from build123d import *

# Parameters (mm, degrees)
SKETCH2_W           = 55
SKETCH2_H           = 115
BOSS_EXTRUDE1_DEPTH = 5
SKETCH5_W           = 50
SKETCH5_H           = 50
SKETCH5_W_2         = 40
SKETCH5_H_2         = 40
SWEEP2_START        = -22.5
SWEEP2_DEPTH        = 50
SWEEP2_2_DEPTH      = 5
SWEEP2_START_2      = 22.5
SWEEP2_3_DEPTH      = 5
SKETCH11_R          = 12.5
CUT_EXTRUDE2_DEPTH  = 25
SKETCH12_R          = 12.5
CUT_EXTRUDE3_DEPTH  = 25
SKETCH13_W          = 2.5
SKETCH13_H          = 115
BOSS_EXTRUDE2_DEPTH = 50
SKETCH15_W          = 2.5
SKETCH15_H          = 115
BOSS_EXTRUDE3_DEPTH = 50
SKETCH14_R          = 7
CUT_EXTRUDE4_DEPTH  = 2185.475051357


# Read off the part's stored shape, not the designer's step: Sweep2
with BuildPart() as part:
    # Sketch2 → Boss-Extrude1 (new body)
    with BuildSketch(Plane(origin=(0, 0, 0), x_dir=(1, 0, 0), z_dir=(0, 1, 0))):
        Rectangle(SKETCH2_W, SKETCH2_H)
    extrude(amount=-BOSS_EXTRUDE1_DEPTH)

    # Sweep1: sweep along a path in Sketch7
    with BuildLine(Plane(origin=(0, 0, 0), x_dir=(0, 0, -1), z_dir=(1, 0, 0))) as sweep1_path:
        Line((-2.5, 0), (-2.5, 1930))
    # Sketch5 → Sweep1 (sweep)
    with BuildSketch(Plane(origin=(0, 0, 0), x_dir=(1, 0, 0), z_dir=(0, 1, 0))):
        with Locations((0, -2.5)):
            Rectangle(SKETCH5_W, SKETCH5_H)
        with Locations((0, -2.5)):
            Rectangle(SKETCH5_W_2, SKETCH5_H_2, mode=Mode.SUBTRACT)
    sweep(path=sweep1_path.line)

    # Sweep2 outline → Sweep2 (add)
    with BuildSketch(Plane.XY.offset(SWEEP2_START)):
        with BuildLine():
            ThreePointArc((125, 2080), (18.933982822, 2036.066017178), (-25, 1930))
            Line((-25, 1930), (-20, 1930))
            ThreePointArc((-20, 1930), (22.469516728, 2032.530483272), (125, 2075))
            Line((125, 2075), (305, 2075))
            Line((305, 2075), (305, 2080))
            Line((305, 2080), (125, 2080))
        make_face()
        with BuildLine():
            ThreePointArc((125, 2035), (50.753787975, 2004.246212025), (20, 1930))
            Line((20, 1930), (25, 1930))
            ThreePointArc((25, 1930), (54.289321881, 2000.710678119), (125, 2030))
            Line((125, 2030), (305, 2030))
            Line((305, 2030), (305, 2035))
            Line((305, 2035), (125, 2035))
        make_face()
    extrude(amount=SWEEP2_DEPTH)

    # Sweep2 2 outline → Sweep2 2 (add)
    with BuildSketch(Plane.XY.offset(SWEEP2_START)):
        with BuildLine():
            ThreePointArc((125, 2075), (22.469516728, 2032.530483272), (-20, 1930))
            Line((-20, 1930), (20, 1930))
            ThreePointArc((20, 1930), (50.753787975, 2004.246212025), (125, 2035))
            Line((125, 2035), (305, 2035))
            Line((305, 2035), (305, 2075))
            Line((305, 2075), (125, 2075))
        make_face()
    extrude(amount=SWEEP2_2_DEPTH)

    # Sweep2 3 outline → Sweep2 3 (add)
    with BuildSketch(Plane.XY.offset(SWEEP2_START_2)):
        with BuildLine():
            ThreePointArc((125, 2075), (22.469516728, 2032.530483272), (-20, 1930))
            Line((-20, 1930), (20, 1930))
            ThreePointArc((20, 1930), (50.753787975, 2004.246212025), (125, 2035))
            Line((125, 2035), (305, 2035))
            Line((305, 2035), (305, 2075))
            Line((305, 2075), (125, 2075))
        make_face()
    extrude(amount=SWEEP2_3_DEPTH)

    # Mirror1: part across plane


with BuildPart() as part_1:
    add(part.part)
    add(part.part.mirror(Plane(origin=(305, 2055, 0), x_dir=(0, 0, 1), z_dir=(1, 0, 0))))

    # Sketch11 → Cut-Extrude2 (cut)
    with BuildSketch(Plane.XZ.offset(-2030)):
        with Locations((395, 2.5)):
            Circle(SKETCH11_R)
    extrude(amount=-CUT_EXTRUDE2_DEPTH, mode=Mode.SUBTRACT)

    # Sketch12 → Cut-Extrude3 (cut)
    with BuildSketch(Plane.XZ.offset(-2030)):
        with Locations((395, 2.5)):
            Circle(SKETCH12_R)
        with Locations(Location((215, 2.5, 0), (0, 0, 180))):
            Circle(SKETCH12_R)
    extrude(amount=-CUT_EXTRUDE3_DEPTH, mode=Mode.SUBTRACT)

    # Sketch13 → Boss-Extrude2 (add)
    with BuildSketch(Plane.XZ.offset(5)):
        with Locations((-26.25, 0)):
            Rectangle(SKETCH13_W, SKETCH13_H)
    extrude(amount=BOSS_EXTRUDE2_DEPTH)

    # Sketch15 → Boss-Extrude3 (add)
    with BuildSketch(Plane.XZ.offset(5)):
        with Locations((636.25, 0)):
            Rectangle(SKETCH15_W, SKETCH15_H)
    extrude(amount=BOSS_EXTRUDE3_DEPTH)

    # Sketch14 → Cut-Extrude4 (cut, through all)
    with BuildSketch(Plane.ZY.offset(27.5)):
        with Locations((-45, -27.5)):
            Circle(SKETCH14_R)
        with Locations((45, -27.5)):
            Circle(SKETCH14_R)
    extrude(amount=-CUT_EXTRUDE4_DEPTH, mode=Mode.SUBTRACT)


solid = part_1.part
The listing builds one solid part. Answer for the finished solid, in the listing's coordinates (mm). A direction names the side the tool comes from. Coordinates: 2 decimals unless noted, no trailing zeros. Loops run counter-clockwise (first coordinate to the right, second up) from the corner with the lowest first, then second, coordinate; pieces in that order, holes last. Notation, with made-up numbers: M 28,42.5 L 34,42.5 A20 cw 34,78.5 Z; hole C 33.25,49 d10. An arc over 180 degrees is marked long. Answer in a Markdown table with one row per item.
1) Determine the mould class of faces 1 (the cylindrical face through (20.11, 2037.23, 2.15)), 2 (the cylindrical face through (21.35, 2031.4, 2.22)), 3 (the flat face through (308, 2030, 2)) for opening direction Y: released by +Y, released by -Y, zero draft, split by the parting line, or undercut.
Answers below:
| item | result |
|---|---|
| face 1 | released by +Y |
| face 2 | undercut |
| face 3 | released by -Y |
2) Find section A-A (y = 999). Determine the outline of the cut face in (x, z), then the cut area to 3 significant figures.
Answers below:
| item | result |
|---|---|
| outline | M -25,-22.5 L 25,-22.5 L 25,27.5 L -25,27.5 Z; M 585,-22.5 L 635,-22.5 L 635,27.5 L 585,27.5 Z; hole M -20,-17.5 L 20,-17.5 L 20,22.5 L -20,22.5 Z; hole M 590,-17.5 L 630,-17.5 L 630,22.5 L 590,22.5 Z |
| area | 1,800 mm^2 |
3) Given pin 1 (20 mm diameter, centred on y = 571.5, z = -7.5, fed in from +X); pin 2 (12 mm diameter, centred on x = 616, z = -3, fed in from +Y); pin 3 (8.5 mm diameter, centred on y = -27.5, z = 45, fed in from -X); pin 4 (3 mm diameter, centred on x = 354, z = 17, fed in from -Y), each flat-ended and moving along its own axis, determine where each tip first touches the part or whether it passes through.
Answers below:
| item | result |
|---|---|
| pin 1 | x = 635 |
| pin 2 | y = 2012.92 |
| pin 3 | through |
| pin 4 | y = 2030 |
4) Find the intervals of material crossed by probe 1 along X at (y, z) = (1484, -8); probe 2 along Y at (x, z) = (-26.6, -45); probe 3 along X at (y, z) = (1209, -19), in increasing order.
Answers below:
| item | result |
|---|---|
| probe 1 | -25 to -20, 20 to 25, 585 to 590, 630 to 635 |
| probe 2 | -55 to -34.5, -20.5 to 0 |
| probe 3 | -25 to 25, 585 to 635 |
5) Find section C-C (x = 527.5). Determine the outline of the cut face in (y, z).
Answers below:
| item | result |
|---|---|
| outline | M 2020.52,-22.5 L 2073.85,-22.5 L 2073.85,27.5 L 2020.52,27.5 Z; hole M 2026.01,-17.5 L 2068.63,-17.5 L 2068.63,22.5 L 2026.01,22.5 Z |
6) Which of the six approach directions +Z, -Z, +X, -X, +Y, -Y give full straight-line access (tool end or side, diameter ignored) to faces 4 (the flat face through (590, 979, 2)), 5 (the flat face through (-8, -3, 57.5)), 6 (the flat face through (635, -30, -1)), 7 (the flat face through (25, 979, 3)), 8 (the flat face through (616, -3, -57.5))?
Answers below:
| item | result |
|---|---|
| face 4 | none |
| face 5 | +Z, +X, -X, +Y, -Y |
| face 6 | +Z, -Z, -Y |
| face 7 | +Z, -Z |
| face 8 | -Z, +X, -X, +Y, -Y |
7) Find section B-B (x = 291). Determine the outline of the cut face in (y, z), then the cut area to 3 significant figures.
Answers below:
| item | result |
|---|---|
| outline | M 2030,-22.5 L 2080,-22.5 L 2080,27.5 L 2030,27.5 Z; hole M 2035,-17.5 L 2075,-17.5 L 2075,22.5 L 2035,22.5 Z |
| area | 900 mm^2 |
